Autodesk Inventor part; units mm, degrees
ref_plane "YZ Plane" through (0, 0, 0) normal (1, 0, 0) x (0, 1, 0)
ref_plane "XZ Plane" through (0, 0, 0) normal (0, 1, 0) x (-1, 0, 0)
ref_plane "XY Plane" through (0, 0, 0) normal (0, 0, 1) x (1, 0, 0)
sketch "Washer Cross Section" plane through (0, 0, 0) normal (0, 1, 0) x (-1, 0, 0)
  circle A0 centre (0, 0) radius 3.3
  dimension "d0" = 6.6
extrude "Washer" add sketch "Washer Cross Section" against normal blind 9.53
sketch "Shoulder Cross Section" plane through (0, 0, 0) normal (0, 1, 0) x (1, 0, 0)
  circle A0 centre (0, 0) radius 5
  dimension "d3" = 10
extrude "Shoulder" add sketch "Shoulder Cross Section" along normal blind 1.6
sketch "Screw Hole Position" plane through (0, 1.6, 0) normal (0, 1, 0) x (1, 0, 0)
  point P0 (0, 0)
  point P1 (0, 0)
hole "Screw Hole" at (0, 1.6, 0) direction (0, -1, 0) diameter 5.08 end through all
properties part number "HSHW-M5-6.6-N" material "Nylon 6/6"
Geometry check sheet. Reference: the model listing, model coordinates, mm. A direction names the side the tool comes from. Coordinates: 2 decimals unless noted, no trailing zeros. Order: outer loops, then holes, each group sorted by start corner. A loop starts at its lowest first (then second) coordinate and runs counter-clockwise, first axis right, second up. Notation, with made-up numbers: M 85.25,23.25 L 93.25,23.25 A19 cw 93.25,40.25 Z; hole C -39.5,-19 d11. An arc over 180 degrees is marked long. Answer as a JSON object with one key per item and string values.
Q1. Scan lines: line 1 (Z direction, x = 0, y = -6.75); line 2 (Z direction, x = 0, y = 0.75); line 3 (Y direction, x = -3.5, z = 0.5). Record each from-to range of solid material in increasing order.
Results are:
{"line 1": "z = -3.3 to -2.54, 2.54 to 3.3", "line 2": "z = -5 to -2.54, 2.54 to 5", "line 3": "y = 0 to 1.6"}
Q2. Cross-section at B-B on z = 0. Record the cut outline in (x, y), and give its area (3 significant figures).
Results are:
{"outline": "M -5,0 L -3.3,0 L -3.3,-9.53 L -2.54,-9.53 L -2.54,1.6 L -5,1.6 Z; M 2.54,-9.53 L 3.3,-9.53 L 3.3,0 L 5,0 L 5,1.6 L 2.54,1.6 Z", "area": "22.4 mm²"}
Q3. Cross-section at D-D on z = -3. Record the cut outline in (x, y).
Results are:
{"outline": "M -4,0 L -1.37,0 L -1.37,-9.53 L 1.37,-9.53 L 1.37,0 L 4,0 L 4,1.6 L -4,1.6 Z"}
Q4. Tool access check on faces 1 (the flat face through (3.3, 0, -1.2)), 2 (the cylindrical face through (-1.08, 0.79, -4.88)). Record the directions out of +Z, -Z, +X, -X, +Y, -Y that give a thin tool (end or side, any length) a straight path to the whole face; none if there is none.
Results are:
{"face 1": "-Y", "face 2": "+Y, -Y"}
Q5. Cross-section at C-C on y = -5.25. Record the cut outline in (x, z).
Results are:
{"outline": "C 0,0 d6.6; hole C 0,0 d5.08"}
Q6. Release check for a two-part mould opening along Z. For faces 3 (the cylindrical face through (2.43, -4.7, 2.23)), 4 (the flat face through (2, 1.6, 2)), 5 (the cylindrical face through (-2.52, -4.04, -0.33)) record: released by +Z, released by -Z, zero draft, split by the parting line, or undercut.
Results are:
{"face 3": "split by the parting line", "face 4": "zero draft", "face 5": "undercut"}
Q7. Cross-section at A-A on x = 0. Record the cut outline in (y, z), and give its area (3 significant figures).
Results are:
{"outline": "M -9.53,-3.3 L 0,-3.3 L 0,-5 L 1.6,-5 L 1.6,-2.54 L -9.53,-2.54 Z; M -9.53,2.54 L 1.6,2.54 L 1.6,5 L 0,5 L 0,3.3 L -9.53,3.3 Z", "area": "22.4 mm²"}
Q8. Depth check by flat-ended pin: pin 1 Ø1 at (x, y) = (0, -4.5) entering from +Z; pin 2 Ø5 at (x, y) = (4, -7) entering from +Z; pin 3 Ø6 at (x, y) = (2, -5.5) entering from -Z. Enter the tip coordinate at first touch or a pass-through.
Results are:
{"pin 1": "stops at z = 3.3", "pin 2": "stops at z = 2.94", "pin 3": "stops at z = -3.3"}
